Verification items for this drawing (mm, ordinates from the low corner). A direction names the side the tool comes from. Round coordinates to 2 decimals unless told otherwise and drop trailing zeros. Loops run counter-clockwise (first coordinate to the right, second up) from the corner with the lowest first, then second, coordinate; pieces in that order, holes last. Notation, with made-up numbers: (77, 21.5) - (85, 21.5) arc R17 cw to (85, 30.5) - close; hole circle Ø7 at (5.5, 55). An arc over 180 degrees is marked (long way). Answer in a Markdown table with one row per item. Add a question column.
(1) Gauge pin test, flat ends, axial feed: pin 1 (10 mm diameter, centred on x = 9.525, y = 9.525, fed in from +Z); pin 2 (2 mm diameter, centred on x = 13.5, z = 10, fed in from +Y); pin 3 (6 mm diameter, centred on y = 11, z = 5, fed in from -X). Record the tip position at first contact, or that the pin passes through.
(2) Cross-section at A-A on x = 11.25. Enter the section's corners in (y, z).
(3) Access from +Z, -Z, +X, -X, +Y, -Y to the whole of each face (thin tool, end or side, straight path). Record for the marked faces 1 and 2.
(4) Thickness scan on line 1 along Z through (x, y) = (1.5, 17.25). Record the ranges inside material, lowest first.
(5) Mould release check, pull along Y, two halves, no side actions. Record for the marked faces 3, 4 and 5: +Y half, -Y half, draft (parallel to the pull), parting line (faces both ways), or undercut.
(6) Cross-section at C-C on y = 4. Enter the section's corners in (x, z).
(7) Cross-section at B-B on y = 7. Enter the section's corners in (x, z).
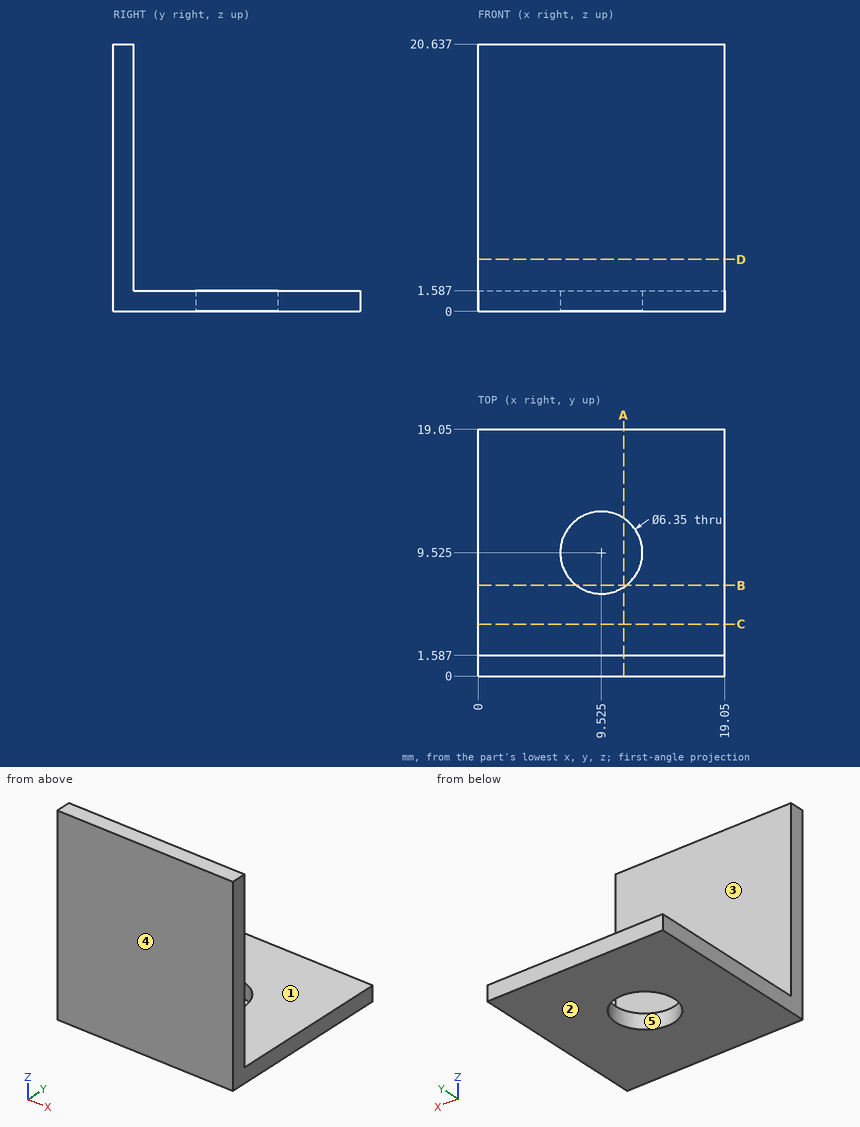
Answers:
| question | item | result |
|---|---|---|
| 1 | pin 1 | stops at z = 1.59 |
| 1 | pin 2 | stops at y = 1.59 |
| 1 | pin 3 | passes through |
| 2 | outline | (0, 0) - (6.86, 0) - (6.86, 1.59) - (1.59, 1.59) - (1.59, 20.64) - (0, 20.64) - close; (12.19, 0) - (19.05, 0) - (19.05, 1.59) - (12.19, 1.59) - close |
| 3 | face 1 | +Z, +X, -X, +Y |
| 3 | face 2 | -Z, +X, -X, +Y, -Y |
| 4 | line 1 | z = 0 to 1.59 |
| 5 | face 3 | +Y half |
| 5 | face 4 | -Y half |
| 5 | face 5 | undercut |
| 6 | outline | (0, 0) - (19.05, 0) - (19.05, 1.59) - (0, 1.59) - close |
| 7 | outline | (0, 0) - (7.6, 0) - (7.6, 1.59) - (0, 1.59) - close; (11.45, 0) - (19.05, 0) - (19.05, 1.59) - (11.45, 1.59) - close |
